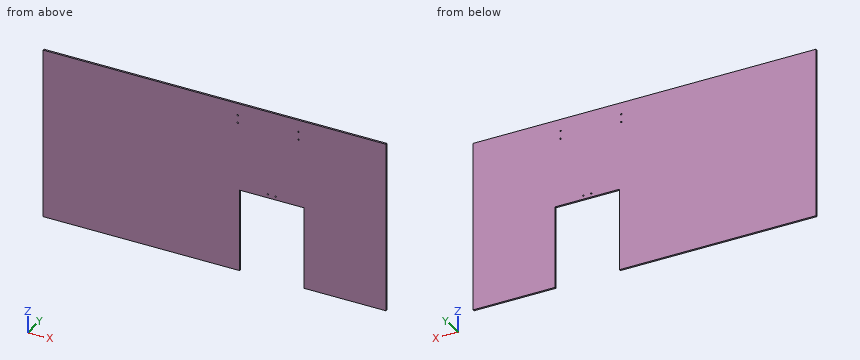
Autodesk Inventor part; units mm, degrees
ref_plane "YZ Plane" through (0, 0, 0) normal (1, 0, 0) x (0, 1, 0)
ref_plane "XZ Plane" through (0, 0, 0) normal (0, 1, 0) x (-1, 0, 0)
ref_plane "XY Plane" through (0, 0, 0) normal (0, 0, 1) x (1, 0, 0)
sketch "Sketch1" plane through (0, 0, 0) normal (0, 1, 0) x (-1, 0, 0)
  line L0 (609.6, 304.8) -> (-609.6, 304.8)
  line L1 (-609.6, 304.8) -> (-609.6, -304.8)
  line L2 (-609.6, -304.8) -> (609.6, -304.8)
  line L3 (609.6, -304.8) -> (609.6, 304.8)
  line L4 (609.6, 304.8) -> (-609.6, -304.8) construction
  line L5 (-609.6, 304.8) -> (609.6, -304.8) construction
  point P0 (0, 0)
  dimension "d0" = 609.6
  dimension "d1" = 1219.2
extrude "Extrusion1" add sketch "Sketch1" along normal blind 6.35
sketch "Sketch2" plane through (0, 6.35, 0) normal (0, 1, 0) x (1, 0, 0)
  line L0 (88.9, 10.16) -> (317.5, 10.16)
  line L1 (317.5, 10.16) -> (317.5, 304.8)
  line L2 (317.5, 304.8) -> (88.9, 304.8)
  line L3 (88.9, 304.8) -> (88.9, 10.16)
  line L4 (88.9, 10.16) -> (317.5, 304.8) construction
  line L5 (317.5, 10.16) -> (88.9, 304.8) construction
  line L6 (609.6, 304.8) -> (-609.6, 304.8)
  line L7 (-609.6, 304.8) -> (-609.6, -304.8)
  line L8 (609.6, -304.8) -> (609.6, 304.8)
  point P0 (0, 0)
  point P1 (203.2, 157.48)
  dimension "d4" = 228.6
  dimension "d5" = 294.64
  dimension "d9" = 292.1
extrude "Extrusion2" cut sketch "Sketch2" against normal up to next
sketch "Sketch3" plane through (0, 6.35, 0) normal (0, 1, 0) x (1, 0, 0)
  circle A0 centre (298.45, -262.1026) radius 2.54
  circle A1 centre (298.45, -234.1626) radius 2.54
  circle A2 centre (82.55, -262.1026) radius 2.54
  circle A3 centre (82.55, -234.1626) radius 2.54
  line L0 (-609.6, -304.8) -> (609.6, -304.8)
  line L1 (609.6, -304.8) -> (609.6, 304.8)
  line L2 (317.5, 304.8) -> (317.5, 10.16)
  circle A4 centre (217.17, -2.54) radius 2.54
  circle A5 centre (189.23, -2.54) radius 2.54
  line L3 (317.5, 10.16) -> (88.9, 10.16)
  line L4 (88.9, 10.16) -> (88.9, 304.8)
  line L5 (88.9, 10.16) -> (317.5, 10.16)
  line L6 (203.2, 10.16) -> (203.2, -2.54) construction
  point P0 (0, 0)
  dimension "d10" = 5.08
  dimension "d14" = 27.94
  dimension "d16" = 215.9
  dimension "d18" = 42.6974
  dimension "d26" = 19.05
  dimension "d27" = 12.7
  dimension "d31" = 27.94
extrude "Extrusion4" cut sketch "Sketch3" against normal up to next
properties part number "Table Top .25 in"
Read the model definition and answer for the solid it produces. Units are mm, in the model's axes. Round coordinates to 2 decimals unless told otherwise and drop trailing zeros. Loops run counter-clockwise (first coordinate to the right, second up) from the corner with the lowest first, then second, coordinate; pieces in that order, holes last.
Q1. Consider probe 1 along Z at (x, y) = (298.45, 1.5); probe 2 along Z at (x, y) = (82.55, 5); probe 3 along Z at (x, y) = (189.23, 4.25). Determine where each line is inside the solid, lowest interval first.
Q2. Section B-B on y = 2.5 is taken. Write down the section's boundary in (x, z).
Q3. Section C-C on x = 121 is taken. Write down the section's boundary in (y, z).
Q4. Section A-A on z = -239.5 is taken. Write down the section's boundary in (x, y), and give its area (3 significant figures).
Q5. Each of these flat-tipped pins is pushed along its axis until it touches: pin 1 (3 mm diameter, centred on x = 82.55, z = 262.1, fed in from -Y); pin 2 (3 mm diameter, centred on x = 251.5, y = 2.5, fed in from -Z). Where does it stop, or does it pass through?
Output:
1. probe 1: z = -10.16 to 231.62, 236.7 to 259.56, 264.64 to 304.8
1. probe 2: z = -304.8 to 231.62, 236.7 to 259.56, 264.64 to 304.8
1. probe 3: z = -10.16 to 0, 5.08 to 304.8
2. outline: (-609.6, -304.8) - (88.9, -304.8) - (88.9, -10.16) - (317.5, -10.16) - (317.5, -304.8) - (609.6, -304.8) - (609.6, 304.8) - (-609.6, 304.8) - close; hole circle Ø5.08 at (82.55, 234.16); hole circle Ø5.08 at (82.55, 262.1); hole circle Ø5.08 at (189.23, 2.54); hole circle Ø5.08 at (217.17, 2.54); hole circle Ø5.08 at (298.45, 234.16); hole circle Ø5.08 at (298.45, 262.1)
3. outline: (0, -10.16) - (6.35, -10.16) - (6.35, 304.8) - (0, 304.8) - close
4. outline: (-609.6, 0) - (88.9, 0) - (88.9, 6.35) - (-609.6, 6.35) - close; (317.5, 0) - (609.6, 0) - (609.6, 6.35) - (317.5, 6.35) - close
4. area: 6,290 mm2
5. pin 1: passes through
5. pin 2: stops at z = -10.16
